Autodesk Inventor part; units mm, degrees
ref_plane "YZ Plane" through (0, 0, 0) normal (1, 0, 0) x (0, 1, 0)
ref_plane "XZ Plane" through (0, 0, 0) normal (0, 1, 0) x (-1, 0, 0)
ref_plane "XY Plane" through (0, 0, 0) normal (0, 0, 1) x (1, 0, 0)
sketch "Skizze1" plane through (0, 0, 0) normal (0, 0, 1) x (1, 0, 0)
  line L0 (-68.016, 1.808) -> (67.584, 1.808)
  line L1 (67.584, 1.808) -> (67.584, -2.192)
  line L2 (67.584, -2.192) -> (-68.016, -2.192)
  line L3 (-68.016, -2.192) -> (-68.016, 1.808)
  line L4 (-68.016, 1.808) -> (67.584, -2.192) construction
  line L5 (67.584, 1.808) -> (-68.016, -2.192) construction
  point P0 (0, 0)
  point P1 (-0.216, -0.192)
  point P2 (-0.216, -0.192)
  dimension "d0" = 135.6
  dimension "d1" = 4
extrude "Extrusion1" add sketch "Skizze1" along normal mid plane 3.25
ref_plane "Arbeitsebene1" through (-68.016, -0.192, 1.625) normal (0, -1, 0) x (1, 0, 0)
sketch "Skizze2" plane through (-68.016, -0.192, 1.625) normal (0, -1, 0) x (1, 0, 0)
  line L0 (0, -3.25) -> (0, 0)
  line L1 (0, -3.25) -> (135.6, -3.25)
  line L2 (0, 0) -> (2.85, 0)
  line L3 (2.85, 0) -> (2.85, -3.25)
  line L4 (2.85, -3.25) -> (0, -3.25)
  line L5 (0, -3.25) -> (0, 0)
  line L6 (0, 0) -> (0, 1.75)
  line L7 (0, 1.75) -> (2.85, 0)
  line L8 (135.6, -3.25) -> (135.6, 0)
  line L9 (135.6, 0) -> (132.75, 0)
  line L10 (132.75, 0) -> (132.75, -3.25)
  line L11 (132.75, -3.25) -> (135.6, -3.25)
  line L12 (135.6, -3.25) -> (135.6, 0)
  line L13 (135.6, 0) -> (135.6, 1.75)
  line L14 (135.6, 1.75) -> (132.75, 0)
  point P0 (68.016, -1.625)
  dimension "d4" = 2.85
  dimension "d5" = 1.75
  dimension "d6" = 2.85
extrude "Extrusion2" add sketch "Skizze2" along normal mid plane 19.7
sketch "Skizze7" plane through (0, 0, 1.625) normal (0, 0, 1) x (1, 0, 0)
  line L0 (64.734, -2.192) -> (-65.166, -2.192)
  line L1 (64.734, 1.808) -> (-65.166, 1.808)
  line L2 (64.734, -2.192) -> (59.734, -2.192)
  line L3 (59.734, -2.192) -> (59.734, 1.808)
  line L4 (59.734, 1.808) -> (64.734, 1.808)
  line L5 (64.734, 1.808) -> (64.734, -2.192)
  line L6 (-65.166, -2.192) -> (-65.166, -10.042)
  line L7 (-65.166, -2.192) -> (-60.166, -2.192)
  line L8 (-60.166, -2.192) -> (-60.166, 1.808)
  line L9 (-60.166, 1.808) -> (-65.166, 1.808)
  line L10 (-65.166, 1.808) -> (-65.166, -2.192)
  line L11 (59.734, 1.808) -> (-60.166, 1.808)
  line L12 (-60.166, 1.808) -> (-60.166, -2.192)
  line L13 (-60.166, -2.192) -> (59.734, -2.192)
  line L14 (59.734, -2.192) -> (59.734, 1.808)
  point P0 (0, 0)
  point P1 (-60.166, 1.808)
  dimension "d27" = 5
  dimension "d28" = 5
extrude "Extrusion7" add sketch "Skizze7" against normal blind 63.25 contours L0 L8 L1 L3
sketch "Skizze8" plane through (-65.166, -2.192, 1.625) normal (0, -1, 0) x (1, 0, 0)
  line L0 (124.9, -3.25) -> (124.9, -63.25)
  line L1 (129.9, 0) -> (0, 0)
  line L2 (124.9, -3.25) -> (119.9, -3.25)
  line L3 (119.9, -3.25) -> (119.9, 0)
  line L4 (119.9, 0) -> (124.9, 0)
  line L5 (124.9, 0) -> (124.9, -3.25)
  line L6 (4.9878, -3.25) -> (9.9878, -3.25)
  line L7 (9.9878, -3.25) -> (9.9878, 0)
  line L8 (9.9878, 0) -> (4.9878, 0)
  line L9 (4.9878, 0) -> (4.9878, -3.25)
  line L10 (119.9, 0) -> (9.9878, 0)
  line L11 (9.9878, 0) -> (9.9878, -58.25)
  line L12 (9.9878, -58.25) -> (119.9, -58.25)
  line L13 (119.9, -58.25) -> (119.9, 0)
  point P0 (65.166, -1.625)
  dimension "d31" = 5
  dimension "d32" = 5
  dimension "d34" = 58.25
extrude "Extrusion8" cut sketch "Skizze8" against normal through all contours L3 L13 L12 L11 L7 L1
ref_plane "Arbeitsebene2" through (-0.222, -2.192, 1.625) normal (1, 0, 0) x (0, 0, -1)
sketch "Skizze9" plane through (-55.1781, -2.192, -56.625) normal (0, 0, 1) x (1, 0, 0)
  circle A0 centre (54.9561, 2.0001) radius 10.8
  point P0 (55.1781, 2.192)
  dimension "d38" = 21.6
extrude "Extrusion9" cut sketch "Skizze9" against normal through all
sketch "Skizze10" plane through (-55.1781, -2.192, -56.625) normal (0, 0, 1) x (1, 0, 0)
  circle A0 centre (54.956, 1.9999) radius 9.4
  circle A1 centre (54.956, 1.9999) radius 11.4
  line L0 (39.8004, -3.1984) -> (71.2174, -3.1984)
  point P0 (55.1781, 2.192)
  point P1 (62.7878, -3.1984)
  point P2 (65.1018, -3.1984)
  point P3 (44.8102, -3.1984)
  point P4 (47.1242, -3.1984)
  dimension "d41" = 18.8
  dimension "d42" = 22.8
extrude "Extrusion10" add sketch "Skizze10" against normal blind 5 contours A0 L0 A1 picked at (65.5795, 2.9069)
properties part number "2025_07_28_Holder_H2_O2_reactor_BOLA_GL14_V0.3"
Here's how the part is built. I have some questions about the finished solid (model axes, mm). A direction names the side the tool comes from. Give positions to 0.01 mm unless a question says otherwise; leave off trailing zeros. Loops run counter-clockwise (first coordinate to the right, second up) from the corner with the lowest first, then second, coordinate; pieces in that order, holes last. Notation, with made-up numbers: M 13,87 L 32,87 A14 cw 32,114 Z; hole C 6.25,72.5 d4. An arc over 180 degrees is marked long. Use one line per item in the form item = value. Start each with the question number.
Q1. If we section it at D-D (x = -43): Write out the boundary of the cut face in (y, z) (3 decimals), then the cut area to 3 significant figures.
Q2. If we section it at B-B (y = 4): Write out the boundary of the cut face in (x, z) (3 decimals), then the cut area to 3 significant figures.
Q3. I need wall thicknesses on line 1 along X through (y, z) = (-1.5, -31.5); line 2 along Y through (x, z) = (-57, -1); line 3 along Z through (x, y) = (-56, 0.5) (3 decimals). Which ranges of each line are inside material? Lowest first, please.
Q4. Which directions (+Z, -Z, +X, -X, +Y, -Y) give clear straight access to the entire face, cutting with the end or side of a thin tool? Please do faces 4 (the flat face through (-67, -10.042, 0)), 5 (the flat face through (-55.178, 0, -27)), 6 (the flat face through (-65.166, -6, 0)).
Q5. Will these pins go through, and if not, where does the flat tip stop? pin 1 Ø3 at (x, y) = (-59.5, 0) entering from +Z (3 decimals); pin 2 Ø1.4 at (x, z) = (-67, 0) entering from +Y; pin 3 Ø10 at (y, z) = (4, -43.5) entering from -X.
Q6. If we section it at A-A (z = -54): Write out the boundary of the cut face in (x, y).
Q7. If we section it at C-C (y = -8): Write out the boundary of the cut face in (x, z) (3 decimals), then the cut area to 3 significant figures.
Q8. Thinking about a two-plate mould opening in X: for faces 1 (the flat face through (64.734, 6, 0)), 2 (the flat face through (59.734, 0, -31)), 3 (the flat face through (-9, -5.39, -59)), which applies, +X half, -X half, draft (parallel to the pull), parting line (faces both ways), or undercut?
Taken from the geometry:
q1.outline = M -2.192,-61.625 L 1.808,-61.625 L 1.808,-56.625 L -2.192,-56.625 Z
q1.area = 20.0 mm^2
q2.outline = M -68.016,-1.625 L -65.166,-1.625 L -65.166,1.625 L -68.016,3.375 Z; M -10.823,-61.625 L -8.636,-61.625 L -8.636,-56.625 L -10.823,-56.625 Z; M 8.191,-61.625 L 10.379,-61.625 L 10.379,-56.625 L 8.191,-56.625 Z; M 64.734,-1.625 L 67.584,-1.625 L 67.584,3.375 L 64.734,1.625 Z
q2.area = 45.4 mm^2
q3.line_1 = -60.17 to -55.18, 54.73 to 59.73
q3.line_2 = -2.19 to 1.81
q3.line_3 = -61.625 to 1.625
q4.face_4 = +Z, -Z, +X, -X, -Y
q4.face_5 = +Z, +Y, -Y
q4.face_6 = +Z, -Z, -Y
q5.pin_1 = 1.625
q5.pin_2 = 9.66
q5.pin_3 = -60.17
q6.outline = M -60.17,-2.19 L -55.18,-2.19 L -55.18,1.81 L -60.17,1.81 Z; M 54.73,-2.19 L 59.73,-2.19 L 59.73,1.81 L 54.73,1.81 Z
q7.outline = M -68.016,-1.625 L -65.166,-1.625 L -65.166,1.625 L -68.016,3.375 Z; M 64.734,-1.625 L 67.584,-1.625 L 67.584,3.375 L 64.734,1.625 Z
q7.area = 23.5 mm^2
q8.face_1 = undercut
q8.face_2 = +X half
q8.face_3 = draft
